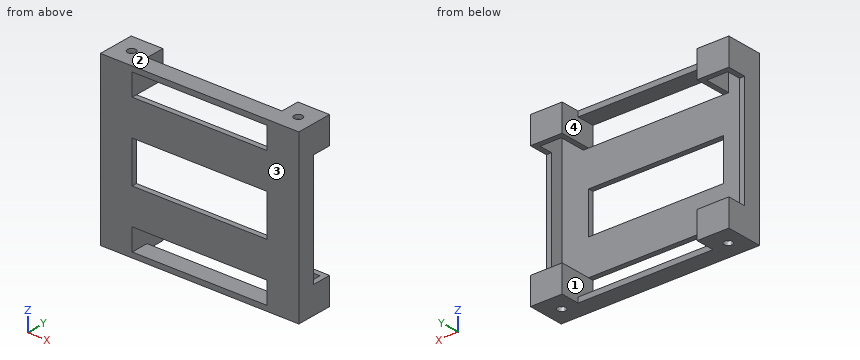
from build123d import *

# Parameters (mm, degrees)
SKETCH1_W                                  = 90
SKETCH1_H                                  = 80
BOSS_EXTRUDE1_DEPTH                        = 2.5
BOSS_EXTRUDE2_DEPTH                        = 13
SKETCH2_3_W                                = 10.2
SKETCH2_3_H                                = 12.6
SKETCH2_3_R                                = 2
BOSS_EXTRUDE3_DEPTH                        = 2
MIRROR1_AT_THE_SECOND_PLANE_COPY_1_DEPTH   = 13
MIRROR1_AT_THE_SECOND_PLANE_COPY_2_SKETC_W = 10.2
MIRROR1_AT_THE_SECOND_PLANE_COPY_2_SKETC_H = 12.6
MIRROR1_AT_THE_SECOND_PLANE_COPY_2_SKETC_R = 2
MIRROR1_AT_THE_SECOND_PLANE_COPY_2_DEPTH   = 2
BOSS_EXTRUDE4_DEPTH                        = 6
BOSS_EXTRUDE4_DEPTH_BACK                   = 2.5
SKETCH4_W                                  = 2.5
SKETCH4_H                                  = 54
SKETCH5_W                                  = 64.6
SKETCH5_H                                  = 10.5
SKETCH5_H_2                                = 20
CUT_EXTRUDE1_DEPTH                         = 64.908215434


with BuildPart() as part:
    # Sketch1 → Boss-Extrude1 (new body)
    with BuildSketch(Plane(origin=(0, 0, 0), x_dir=(1, 0, 0), z_dir=(0, 1, 0))):
        Rectangle(SKETCH1_W, SKETCH1_H)
    extrude(amount=BOSS_EXTRUDE1_DEPTH)

    # Sketch2 → Boss-Extrude2 (add)
    with BuildSketch(Plane.XY.offset(40)):
        Polygon((-45, 15.1), (-34.8, 15.1), (-34.8, 2.5), (-32.3, 2.5), (-32.3, 17.6), (-47.5, 17.6), (-47.5, 0), (-45, 0), (-45, 2.5), align=None)
    boss_extrude2 = extrude(amount=-BOSS_EXTRUDE2_DEPTH)

    # Sketch2<3> → Boss-Extrude3 (add)
    with BuildSketch(Plane.XY.offset(40)):
        with Locations((-39.9, 8.8)):
            Rectangle(SKETCH2_3_W, SKETCH2_3_H)
        with Locations((-39.9, 8.8)):
            Circle(SKETCH2_3_R, mode=Mode.SUBTRACT)
    boss_extrude3 = extrude(amount=-BOSS_EXTRUDE3_DEPTH)

    # Mirror1: Boss-Extrude2, Boss-Extrude3 across plane
    add(boss_extrude2.mirror(Plane.XY))
    add(boss_extrude3.mirror(Plane.XY))

    # Mirror1 at the second plane: Boss-Extrude2, Boss-Extrude3 across plane
    add(boss_extrude2.mirror(Plane(origin=(0, 0, 0), x_dir=(0, 0, 1), z_dir=(1, 0, 0))))
    add(boss_extrude3.mirror(Plane(origin=(0, 0, 0), x_dir=(0, 0, 1), z_dir=(1, 0, 0))))

    # Mirror1 at the second plane copy 1 sketc → Mirror1 at the second plane copy 1 (add)
    with BuildSketch(Plane(origin=(0, 0, -40), x_dir=(-1, 0, 0), z_dir=(0, 0, -1))):
        Polygon((-45, 15.1), (-34.8, 15.1), (-34.8, 2.5), (-32.3, 2.5), (-32.3, 17.6), (-47.5, 17.6), (-47.5, 0), (-45, 0), (-45, 2.5), align=None)
    extrude(amount=-MIRROR1_AT_THE_SECOND_PLANE_COPY_1_DEPTH)

    # Mirror1 at the second plane copy 2 sketc → Mirror1 at the second plane copy 2 (add)
    with BuildSketch(Plane(origin=(0, 0, -40), x_dir=(-1, 0, 0), z_dir=(0, 0, -1))):
        with Locations((-39.9, 8.8)):
            Rectangle(MIRROR1_AT_THE_SECOND_PLANE_COPY_2_SKETC_W, MIRROR1_AT_THE_SECOND_PLANE_COPY_2_SKETC_H)
        with Locations((-39.9, 8.8)):
            Circle(MIRROR1_AT_THE_SECOND_PLANE_COPY_2_SKETC_R, mode=Mode.SUBTRACT)
    extrude(amount=-MIRROR1_AT_THE_SECOND_PLANE_COPY_2_DEPTH)

    # Sketch4 → Boss-Extrude4 (add, two sides: drawn at the far end of the back side and taken through both)
    with BuildSketch(Plane(origin=(0, 2.5, 0), x_dir=(1, 0, 0), z_dir=(0, 1, 0)).offset(-BOSS_EXTRUDE4_DEPTH_BACK)):
        Polygon((32.3, 37.5), (32.3, 40), (-32.3, 40), (-32.3, 37.5), (-29.8, 37.5), (29.8, 37.5), align=None)
        Polygon((32.3, -37.5), (32.3, -40), (-32.3, -40), (-32.3, -37.5), (-29.8, -37.5), (29.8, -37.5), align=None)
        with Locations((46.25, 0)):
            Rectangle(SKETCH4_W, SKETCH4_H)
        with Locations((-46.25, 0)):
            Rectangle(SKETCH4_W, SKETCH4_H)
    extrude(amount=BOSS_EXTRUDE4_DEPTH + BOSS_EXTRUDE4_DEPTH_BACK)

    # Sketch5 → Cut-Extrude1 (cut, through all)
    with BuildSketch(Plane(origin=(0, 2.5, 0), x_dir=(1, 0, 0), z_dir=(0, 1, 0))):
        with Locations((0, -32.25)):
            Rectangle(SKETCH5_W, SKETCH5_H)
        with Locations((0, 32.25)):
            Rectangle(SKETCH5_W, SKETCH5_H)
        Rectangle(SKETCH5_W, SKETCH5_H_2)
    extrude(amount=-CUT_EXTRUDE1_DEPTH, mode=Mode.SUBTRACT)


solid = part.part
Model file for the job. Use its own axes, mm. Face numbers are marked on the shaded views. Give positions to 0.01 mm unless a question says otherwise; leave off trailing zeros. Loops run counter-clockwise (first coordinate to the right, second up) from the corner with the lowest first, then second, coordinate; pieces in that order, holes last.
Item 1: Drill centre lines: line 1 along X through (y, z) = (12, 30); line 2 along Z through (x, y) = (7.5, 5.75); line 3 along Z through (x, y) = (41.5, 13.25). Where is each one in solid material? Low to high.
Check values:
line 1: x = -47.5 to -45, -34.8 to -32.3, 32.3 to 34.8, 45 to 47.5
line 2: z = -40 to -37.5, 37.5 to 40
line 3: z = -40 to -38, 38 to 40
Item 2: Mould opens along Z. For the marked faces 1, 2, 3 and 4 say: +Z half, -Z half, draft (parallel to the pull), parting line (faces both ways), or undercut.
Check values:
face 1: undercut
face 2: +Z half
face 3: draft
face 4: undercut
Item 3: Drop flat-ended pins along their axis: P1, Ø1.2, axis at x = -46.5, z = 0, coming from the +Y side; P2, Ø1.5, axis at x = -33, z = 24.5, coming from the +Y side. Give the stop position or say it passes through.
Check values:
P1: stops at y = 8.5
P2: stops at y = 2.5
Item 4: Slice it at D-D (z = 20). Write the cut outline in (x, y), plus the area to 4 significant figures.
Check values:
outline: (-47.5, 0) - (47.5, 0) - (47.5, 8.5) - (45, 8.5) - (45, 2.5) - (-45, 2.5) - (-45, 8.5) - (-47.5, 8.5) - close
area: 267.5 mm2
Item 5: Slice it at C-C (x = -39.9). Write the cut outline in (y, z), plus the area to 3 significant figures.
Check values:
outline: (0, -40) - (6.8, -40) - (6.8, -38) - (2.5, -38) - (2.5, 38) - (6.8, 38) - (6.8, 40) - (0, 40) - close; (10.8, -40) - (17.6, -40) - (17.6, -27) - (15.1, -27) - (15.1, -38) - (10.8, -38) - close; (10.8, 38) - (15.1, 38) - (15.1, 27) - (17.6, 27) - (17.6, 40) - (10.8, 40) - close
area: 299 mm2
Item 6: Slice it at A-A (x = 11). Write the cut outline in (y, z), plus the area to 4 significant figures.
Check values:
outline: (0, -40) - (8.5, -40) - (8.5, -37.5) - (0, -37.5) - close; (0, -27) - (2.5, -27) - (2.5, -10) - (0, -10) - close; (0, 10) - (2.5, 10) - (2.5, 27) - (0, 27) - close; (0, 37.5) - (8.5, 37.5) - (8.5, 40) - (0, 40) - close
area: 127.5 mm2
Item 7: Slice it at B-B (y = 1.25). Write the cut outline in (x, z).
Check values:
outline: (-47.5, -40) - (47.5, -40) - (47.5, 40) - (-47.5, 40) - close; hole (-32.3, -37.5) - (32.3, -37.5) - (32.3, -27) - (-32.3, -27) - close; hole (-32.3, -10) - (32.3, -10) - (32.3, 10) - (-32.3, 10) - close; hole (-32.3, 27) - (32.3, 27) - (32.3, 37.5) - (-32.3, 37.5) - close
